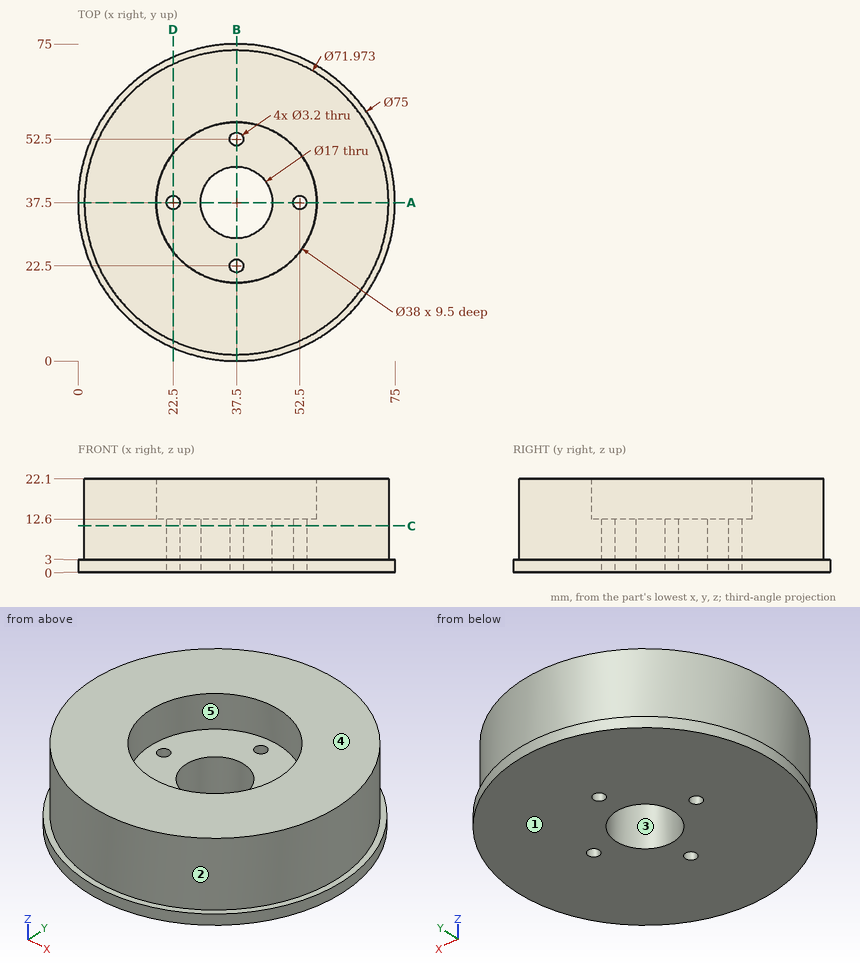
Verification items for this drawing (mm, ordinates from the low corner). A direction names the side the tool comes from. Round coordinates to 2 decimals unless told otherwise and drop trailing zeros. Write each loop counter-clockwise with the first axis right and the second up, starting at its lowest first coordinate (ties: lowest second). Pieces come first, ordered by that corner, then holes. Notation, with made-up numbers: (71.5, 24.5) - (129.5, 24.5) arc R10 ccw to (129.5, 35.5) - close; hole circle Ø3 at (73, 50). An arc over 180 degrees is marked (long way). One line per item, written item: value.
1. Scan lines: L1, parallel to Y at x = 37.5, z = 5.5; L2, parallel to Z at x = 32.5, y = 55; L3, parallel to Y at x = 40.5, z = 19. Record each from-to range of solid material in increasing order.
The answers:
L1: y = 1.51 to 20.9, 24.1 to 29, 46 to 50.9, 54.1 to 73.49
L2: z = 0 to 12.6
L3: y = 1.64 to 18.74, 56.26 to 73.36
2. Cross-section at A-A on y = 37.5. Record the boundary of the cut face in (x, z).
The answers:
outline: (0, 0) - (20.9, 0) - (20.9, 12.6) - (18.5, 12.6) - (18.5, 22.1) - (1.51, 22.1) - (1.51, 3) - (0, 3) - close; (24.1, 0) - (29, 0) - (29, 12.6) - (24.1, 12.6) - close; (46, 0) - (50.9, 0) - (50.9, 12.6) - (46, 12.6) - close; (54.1, 0) - (75, 0) - (75, 3) - (73.49, 3) - (73.49, 22.1) - (56.5, 22.1) - (56.5, 12.6) - (54.1, 12.6) - close
3. Depth check by flat-ended pin: pin 1 Ø4 at (x, y) = (37.5, 22.5) entering from +Z; pin 2 Ø1 at (x, z) = (19, 12) entering from +Y; pin 3 Ø1 at (x, z) = (10.5, 14) entering from -Y. Enter the tip coordinate at first touch or a pass-through.
The answers:
pin 1: stops at z = 12.6
pin 2: stops at y = 68.66
pin 3: stops at y = 13.15
4. Set-up check for the marked faces 4 and 5: record each of +Z, -Z, +X, -X, +Y, -Y from which the full face is reachable in a straight line by a thin tool's end or side.
The answers:
face 4: +Z, +X, -X, +Y, -Y
face 5: +Z
5. Cross-section at C-C on z = 11. Record the boundary of the cut face in (x, y), and give its area (3 significant figures).
The answers:
outline: circle Ø71.97 at (37.5, 37.5); hole circle Ø3.2 at (22.5, 37.5); hole circle Ø17 at (37.5, 37.5); hole circle Ø3.2 at (37.5, 22.5); hole circle Ø3.2 at (37.5, 52.5); hole circle Ø3.2 at (52.5, 37.5)
area: 3,810 mm^2
6. Mould release check, pull along Y, two halves, no side actions. Record for the marked faces 1, 2 and 3: released by +Y, released by -Y, zero draft, split by the parting line, or undercut.
The answers:
face 1: zero draft
face 2: split by the parting line
face 3: undercut
7. Cross-section at D-D on x = 22.5. Record the boundary of the cut face in (y, z).
The answers:
outline: (3.13, 0) - (35.9, 0) - (35.9, 12.6) - (25.84, 12.6) - (25.84, 22.1) - (4.79, 22.1) - (4.79, 3) - (3.13, 3) - close; (39.1, 0) - (71.87, 0) - (71.87, 3) - (70.21, 3) - (70.21, 22.1) - (49.16, 22.1) - (49.16, 12.6) - (39.1, 12.6) - close
